Model file for the job. Use its own axes, mm. A direction names the side the tool comes from. Coordinates: 2 decimals unless noted, no trailing zeros. Write each loop counter-clockwise with the first axis right and the second up, starting at its lowest first coordinate (ties: lowest second). Pieces come first, ordered by that corner, then holes. Notation, with made-up numbers: M 19.5,89.25 L 32.5,89.25 A13 cw 32.5,100.25 Z; hole C 13.5,68 d7. An arc over 180 degrees is marked long. Answer in a Markdown table with one row per item. Add a question column.
```python
from build123d import *

# Parameters (mm, degrees)
SKETCH_1_R          = 1.6
EXTRUDE_1_DEPTH     = 3
CUT_EXTRUDE_1_DEPTH = 1


with BuildPart() as part:
    # 草图1 → 凸台-拉伸1 (new body)
    with BuildSketch(Plane.XY.offset(3)):
        with BuildLine():
            Line((291.102941136, 60.850305737), (291.076707349, 16.850305738))
            ThreePointArc((291.076707349, 16.850305738), (291.954101097, 14.728512603), (294.07484648, 13.848589358))
            Line((294.07484648, 13.848589358), (338.074844131, 13.822355573))
            ThreePointArc((338.074844131, 13.822355573), (340.196637266, 14.699749321), (341.07656051, 16.820494704))
            Line((341.07656051, 16.820494704), (341.102794297, 60.820495366))
            ThreePointArc((341.102794297, 60.820495366), (340.22540099, 62.942287436), (338.104656671, 63.822210239))
            Line((338.104656671, 63.822210239), (294.104656671, 63.848444025))
            ThreePointArc((294.104656671, 63.848444025), (291.982864133, 62.971050524), (291.102941136, 60.850305737))
        make_face()
        with Locations(Location((338.076632755, 16.822283328, 0), (0, 0, 180))):
            Circle(SKETCH_1_R, mode=Mode.SUBTRACT)
        with Locations(Location((294.102868048, 60.848517113, 0), (0, 0, 180))):
            Circle(SKETCH_1_R, mode=Mode.SUBTRACT)
        with Locations(Location((338.102868048, 60.822283989, 0), (0, 0, 180))):
            Circle(SKETCH_1_R, mode=Mode.SUBTRACT)
        with Locations(Location((294.076635104, 16.848517113, 0), (0, 0, 180))):
            Circle(SKETCH_1_R, mode=Mode.SUBTRACT)
        with Locations(Location((316.111204471, 29.315652621, 0), (0, 0, 180))):
            Circle(SKETCH_1_R, mode=Mode.SUBTRACT)
        with Locations(Location((316.090486738, 48.315652621, 0), (0, 0, 180))):
            Circle(SKETCH_1_R, mode=Mode.SUBTRACT)
        Polygon((303.43545239, 46.035704845), (328.682343893, 46.020652083), (328.673787658, 31.669910181), (303.426896156, 31.684962944), align=None, mode=Mode.SUBTRACT)
    extrude(amount=-EXTRUDE_1_DEPTH)

    # 草图2 → 切除-拉伸1 (cut)
    with BuildSketch(Plane.XY.offset(3)):
        with BuildLine():
            Line((315.174630784, 58.972726271), (314.86052822, 58.972726271))
            add(Edge.make_bspline(
                [(314.86052822, 58.972726271), (314.869037771, 59.007958755), (314.885673246, 59.07683538), (314.92037082, 59.17524264), (314.958170075, 59.268366162), (315.003559179, 59.354462236), (315.053067934, 59.435261138), (315.109790655, 59.508930263), (315.171110378, 59.577343228), (315.238935327, 59.638056466), (315.310063989, 59.693034195), (315.385498608, 59.739909252), (315.463721502, 59.780233405), (315.545274635, 59.813453637), (315.630400807, 59.838479161), (315.71833043, 59.856635966), (315.80929393, 59.868427081), (315.871041521, 59.869577844), (315.902395207, 59.870162169)],
                knots=[0, 0, 0, 0, 1.162005537, 2.271625781, 3.343758855, 4.383309926, 5.390229558, 6.379919256, 7.361854164, 8.333198761, 9.295911338, 10.242430842, 11.177959212, 12.116337295, 13.062827104, 14.020064771, 14.994644689, 16, 16, 16, 16], degree=3))
            add(Edge.make_bspline(
                [(315.902395207, 59.870162169), (315.948077949, 59.868782938), (316.03844696, 59.866054563), (316.171210007, 59.841140127), (316.299236826, 59.801714994), (316.421126074, 59.747241267), (316.534344507, 59.680053954), (316.635080693, 59.600089217), (316.721969204, 59.508889915), (316.794863582, 59.408157351), (316.851938581, 59.300501842), (316.894024954, 59.189701685), (316.919646635, 59.076019713), (316.922967192, 58.999262434), (316.924630784, 58.960807201)],
                knots=[0, 0, 0, 0, 1.083050992, 2.142477498, 3.193116406, 4.255571735, 5.30263384, 6.308962982, 7.297363603, 8.282367274, 9.249857812, 10.179914175, 11.08814088, 12, 12, 12, 12], degree=3))
            add(Edge.make_bspline(
                [(316.924630784, 58.960807201), (316.923467193, 58.923800406), (316.921190226, 58.851383852), (316.90185652, 58.745662354), (316.869320257, 58.646020754), (316.824250495, 58.552039592), (316.765908945, 58.464314752), (316.695236248, 58.382648861), (316.611733586, 58.306679703), (316.548454648, 58.26316023), (316.515876778, 58.240755117)],
                knots=[0, 0, 0, 0, 1.024540389, 2.004866551, 2.965041327, 3.920577974, 4.882998113, 5.874504559, 6.905732034, 8, 8, 8, 8], degree=3))
            add(Edge.make_bspline(
                [(316.515876778, 58.240755117), (316.553108532, 58.222776946), (316.626875406, 58.187156988), (316.727425936, 58.117301231), (316.818703811, 58.036644883), (316.86960753, 57.97370223), (316.895183669, 57.942077233)],
                knots=[0, 0, 0, 0, 1.015518401, 2.012035669, 3.001164323, 4, 4, 4, 4], degree=3))
            add(Edge.make_bspline(
                [(316.895183669, 57.942077233), (316.912025011, 57.919019481), (316.945431907, 57.873281565), (316.986667441, 57.799745139), (317.024076555, 57.725393649), (317.053226774, 57.648234243), (317.075800641, 57.56916123), (317.091936674, 57.488038834), (317.101960814, 57.404800811), (317.103396366, 57.348488331), (317.104117964, 57.320182201)],
                knots=[0, 0, 0, 0, 1.025084078, 2.033381695, 3.024893161, 4.013698104, 4.991890475, 5.976764909, 6.982997093, 8, 8, 8, 8], degree=3))
            add(Edge.make_bspline(
                [(317.104117964, 57.320182201), (317.10232345, 57.27117248), (317.098742868, 57.173383678), (317.066738794, 57.028908956), (317.017125553, 56.887683454), (316.946668617, 56.752608615), (316.860801108, 56.626228234), (316.758643784, 56.513151925), (316.641357376, 56.41595332), (316.510551727, 56.334743092), (316.368834598, 56.26982517), (316.217259006, 56.224767727), (316.058008952, 56.195421727), (315.948801655, 56.192274859), (315.893280624, 56.190674989)],
                knots=[0, 0, 0, 0, 0.955779014, 1.907060117, 2.875433937, 3.871313158, 4.872415639, 5.851225146, 6.836215519, 7.83643374, 8.849228613, 9.86973379, 10.916971861, 12, 12, 12, 12], degree=3))
            add(Edge.make_bspline(
                [(315.893280624, 56.190674989), (315.855861324, 56.191543202), (315.782232618, 56.193251557), (315.67398912, 56.204930158), (315.570667421, 56.226260163), (315.472127823, 56.254963468), (315.378282786, 56.291355211), (315.289418681, 56.336673909), (315.204988788, 56.389985411), (315.125789837, 56.451918998), (315.051831269, 56.521200338), (314.985078545, 56.599059348), (314.924418752, 56.684056752), (314.871476113, 56.777179808), (314.82383916, 56.877225066), (314.784658204, 56.985473564), (314.750172635, 57.100957586), (314.734139171, 57.181435326), (314.725912835, 57.222726271)],
                knots=[0, 0, 0, 0, 1.048658725, 2.063410685, 3.046034179, 4.001477787, 4.936774919, 5.862367409, 6.792675028, 7.730719943, 8.675894397, 9.627829632, 10.600096036, 11.597688215, 12.626045268, 13.701542398, 14.82072376, 16, 16, 16, 16], degree=3))
            Line((314.725912835, 57.222726271), (315.040015399, 57.222726271))
            add(Edge.make_bspline(
                [(315.040015399, 57.222726271), (315.048198691, 57.195777258), (315.064115904, 57.143359086), (315.091210202, 57.067918781), (315.122078474, 56.998760727), (315.155193032, 56.935377606), (315.189971478, 56.877145203), (315.228886403, 56.825603334), (315.269055549, 56.778488132), (315.299334902, 56.75194352), (315.314154021, 56.738952233)],
                knots=[0, 0, 0, 0, 1.198163088, 2.33053128, 3.407730985, 4.417276592, 5.372219308, 6.28897303, 7.162600585, 8, 8, 8, 8], degree=3))
            add(Edge.make_bspline(
                [(315.314154021, 56.738952233), (315.333750598, 56.723843899), (315.372883261, 56.693673867), (315.436651492, 56.655172239), (315.503716378, 56.621811213), (315.575531052, 56.596327518), (315.650545823, 56.574749857), (315.729973188, 56.560629338), (315.813112405, 56.550941166), (315.869880168, 56.550086235), (315.898889598, 56.549649348)],
                knots=[0, 0, 0, 0, 0.946170439, 1.889420265, 2.845303464, 3.807233317, 4.801018734, 5.828864929, 6.890507805, 8, 8, 8, 8], degree=3))
            add(Edge.make_bspline(
                [(315.898889598, 56.549649348), (315.931643101, 56.550265253), (315.995689748, 56.551469603), (316.089144607, 56.56254531), (316.178052055, 56.578675723), (316.26142498, 56.603588706), (316.340355488, 56.634369558), (316.413737137, 56.673017963), (316.482533244, 56.718362685), (316.545862649, 56.769901843), (316.602808157, 56.826323338), (316.65294767, 56.885336409), (316.695572331, 56.946692239), (316.729955909, 57.01073036), (316.75710646, 57.077185589), (316.77558966, 57.146244418), (316.788441175, 57.217341684), (316.789487788, 57.265670653), (316.790015399, 57.290033964)],
                knots=[0, 0, 0, 0, 1.217147791, 2.380027433, 3.494444702, 4.572153297, 5.609568379, 6.639424714, 7.649109417, 8.668170816, 9.669597737, 10.625200337, 11.543417969, 12.441394052, 13.322311151, 14.205496177, 15.095365482, 16, 16, 16, 16], degree=3))
            add(Edge.make_bspline(
                [(316.790015399, 57.290033964), (316.788485098, 57.322645302), (316.785432109, 57.387705711), (316.76212353, 57.483423285), (316.723784666, 57.575646697), (316.670112154, 57.662802487), (316.604776426, 57.743578389), (316.528411519, 57.815649871), (316.440383291, 57.875119963), (316.359363422, 57.916208619), (316.287598265, 57.944245694), (316.226182881, 57.962920659), (316.157426277, 57.978734314), (316.082159928, 57.993446586), (315.999816712, 58.005967934), (315.910486274, 58.01640975), (315.814150512, 58.024764791), (315.747459346, 58.028495886), (315.713092323, 58.030418579)],
                knots=[0, 0, 0, 0, 1.07054697, 2.135767047, 3.216561865, 4.33974944, 5.486079747, 6.621378074, 7.775625952, 8.963672916, 9.598146892, 10.304877434, 11.070270905, 11.915000392, 12.823868403, 13.805723172, 14.86925407, 16, 16, 16, 16], degree=3))
            Line((315.713092323, 58.030418579), (315.713092323, 58.389392938))
            add(Edge.make_bspline(
                [(315.713092323, 58.389392938), (315.756393488, 58.390127742), (315.841209835, 58.391567042), (315.96510414, 58.408975052), (316.083577452, 58.43305568), (316.194004194, 58.469940872), (316.294652907, 58.512781169), (316.381972509, 58.562633379), (316.454739656, 58.618048128), (316.512600728, 58.679880737), (316.556129957, 58.746195785), (316.587956754, 58.815312442), (316.60675708, 58.887836503), (316.609266747, 58.937331171), (316.61052822, 58.962209444)],
                knots=[0, 0, 0, 0, 1.321986639, 2.589447074, 3.816329219, 5.01088745, 6.139805852, 7.153945165, 8.075214402, 8.924034688, 9.728124013, 10.488707548, 11.240355623, 12, 12, 12, 12], degree=3))
            add(Edge.make_bspline(
                [(316.61052822, 58.962209444), (316.610113809, 58.980487189), (316.609289358, 59.016849897), (316.59889208, 59.069974965), (316.583268039, 59.121475911), (316.56178831, 59.171133721), (316.533038111, 59.218603995), (316.498632125, 59.264291444), (316.457664024, 59.307935223), (316.410718577, 59.348615543), (316.360306772, 59.38738478), (316.305056997, 59.420298417), (316.246635123, 59.448443479), (316.184976468, 59.471652981), (316.119880938, 59.489112269), (316.05165438, 59.501648111), (315.980166696, 59.509485766), (315.931394964, 59.510614181), (315.906601938, 59.51118781)],
                knots=[0, 0, 0, 0, 0.884392785, 1.759457502, 2.611959086, 3.489218968, 4.37281399, 5.2945488, 6.255912374, 7.266815255, 8.301784654, 9.332968512, 10.37626691, 11.440494194, 12.520033166, 13.637162961, 14.798855837, 16, 16, 16, 16], degree=3))
            add(Edge.make_bspline(
                [(315.906601938, 59.51118781), (315.86675027, 59.509796448), (315.788910694, 59.507078794), (315.676695777, 59.483275781), (315.572376443, 59.445297697), (315.492637776, 59.399964678), (315.433755202, 59.355214244), (315.391678264, 59.316131858), (315.350357753, 59.272699034), (315.312512076, 59.222240659), (315.2742381, 59.168173868), (315.239393538, 59.107750187), (315.205533846, 59.042545793), (315.185131296, 58.996450158), (315.174630784, 58.972726271)],
                knots=[0, 0, 0, 0, 1.472543308, 2.876219568, 4.221790263, 5.565193594, 6.249813518, 6.953379497, 7.687249741, 8.463570142, 9.283606569, 10.136032583, 11.040678096, 12, 12, 12, 12], degree=3))
        make_face()
    extrude(amount=-CUT_EXTRUDE_1_DEPTH, mode=Mode.SUBTRACT)


solid = part.part
```
1) Slice it at D-D (x = 327.5). Give the cut face in (y, z), then the cut area to 3 significant figures.
2) Slice it at C-C (z = 1). Give the cut face in (x, y).
3) Slice it at A-A (x = 337.5). Give the cut face in (y, z).
4) Slice it at B-B (y = 39). Give the cut face in (x, z), then the cut area to 3 significant figures.
5) Drill centre lines: probe 1 along X at (y, z) = (38, 0.65); probe 2 along Y at (x, z) = (311, 0.6); probe 3 along Y at (x, z) = (339, 1.55). Where is each one in solid material? Low to high.
6) Two-plate mould, pull along Y, no slides. Class faces 3 (the face through (340.173, 14.677, 1.521)), 4 (the face through (295.675, 16.778, 1.521)), 5 (the face through (315.7, 50.3, 0)): released by +Y, released by -Y, zero draft, split by the parting line, or undercut.
7) Which spindle directions (+Z, -Z, +X, -X, +Y, -Y) get a long thin tool onto all of the face, cutting with end or side? Do faces 1 (the face through (295.7, 60.78, 1.52)), 2 (the face through (316, 58.2, 2)). Say none if no direction does.
8) Flat gauge pins, fed straight in: pin 1 Ø1.5 at (y, z) = (42.5, 2) entering from +X; pin 2 Ø1.5 at (x, z) = (316.5, 2) entering from -Y. Where does each tip first touch, or does it go through?
Ans:
| question | item | result |
|---|---|---|
| 1 | outline | M 13.83,0 L 31.67,0 L 31.67,3 L 13.83,3 Z; M 46.02,0 L 63.83,0 L 63.83,3 L 46.02,3 Z |
| 1 | area | 107 mm2 |
| 2 | outline | M 291.08,16.85 A3 ccw 294.07,13.85 L 338.07,13.82 A3 ccw 341.08,16.82 L 341.1,60.82 A3 ccw 338.1,63.82 L 294.1,63.85 A3 ccw 291.1,60.85 Z; hole C 294.08,16.85 d3.2; hole C 294.1,60.85 d3.2; hole M 303.43,31.68 L 328.67,31.67 L 328.68,46.02 L 303.44,46.04 Z; hole C 316.09,48.32 d3.2; hole C 316.11,29.32 d3.2; hole C 338.08,16.82 d3.2; hole C 338.1,60.82 d3.2 |
| 3 | outline | M 13.82,0 L 15.33,0 L 15.33,3 L 13.82,3 Z; M 18.31,0 L 59.34,0 L 59.34,3 L 18.31,3 Z; M 62.3,0 L 63.82,0 L 63.82,3 L 62.3,3 Z |
| 4 | outline | M 291.09,0 L 303.43,0 L 303.43,3 L 291.09,3 Z; M 328.68,0 L 341.09,0 L 341.09,3 L 328.68,3 Z |
| 4 | area | 74.3 mm2 |
| 5 | probe 1 | x = 291.09 to 303.43, 328.68 to 341.09 |
| 5 | probe 2 | y = 13.84 to 31.68, 46.03 to 63.84 |
| 5 | probe 3 | y = 13.97 to 15.52, 18.13 to 59.5, 62.15 to 63.68 |
| 6 | face 3 | released by -Y |
| 6 | face 4 | undercut |
| 6 | face 5 | zero draft |
| 7 | face 1 | +Z, -Z |
| 7 | face 2 | +Z |
| 8 | pin 1 | stops at x = 341.09 |
| 8 | pin 2 | stops at y = 13.83 |
